Check sheet for the modelled part. Datum: model origin and axes. Units: mm. Face numbers are marked on the shaded views. Coordinates: 2 decimals unless noted, no trailing zeros. Loops run counter-clockwise (first coordinate to the right, second up) from the corner with the lowest first, then second, coordinate; pieces in that order, holes last. Notation, with made-up numbers: M 10,4 L 25,4 A27 cw 25,34 Z; hole C 37,-39.75 d7. An arc over 180 degrees is marked long. Use CSV: the item, a comma, the result in double quotes. Start each with the question number.
(1) Section check C-C on y = 61. Record the cut outline in (x, z), and give its area (3 significant figures).
(2) Section check A-A on z = 0. Record the cut outline in (x, y), and give its area (3 significant figures).
(3) Draft check along X on the marked faces 1, 2 and 3. Enter one of: pulls with the +X half, pulls with the -X half, needs draft (parallel to the pull), parting line crosses it, or undercut.
(4) Go/stop test with flat-tipped pins: pin 1 Ø4 at (y, z) = (-13.5, -33) entering from -X; pin 2 Ø4 at (y, z) = (-46, 34.5) entering from -X; pin 3 Ø4 at (y, z) = (-39.5, 39) entering from +X. Record where each tip stops, or that it passes through.
(5) Scan lines: line 1 (Z direction, x = 0, y = 8); line 2 (Z direction, x = -20, y = 9.5). Record each from-to range of solid material in increasing order.
(6) Section check B-B on x = 0. Record the cut outline in (y, z), and give its area (3 significant figures).
Autodesk Inventor part; units mm, degrees
ref_plane "YZ Plane" through (0, 0, 0) normal (1, 0, 0) x (0, 1, 0)
ref_plane "XZ Plane" through (0, 0, 0) normal (0, 1, 0) x (-1, 0, 0)
ref_plane "XY Plane" through (0, 0, 0) normal (0, 0, 1) x (1, 0, 0)
sketch "Sketch1" plane through (0, 0, 0) normal (0, 0, 1) x (1, 0, 0)
  line L0 (-50, 88.8965) -> (-25, 88.8965)
  line L1 (-25, 88.8965) -> (-25, -61.1035)
  line L2 (-25, -61.1035) -> (-50, -61.1035)
  line L3 (-50, -61.1035) -> (-50, 88.8965)
  line L4 (0, 88.8965) -> (0, -88.8965)
  point P0 (0, 0)
  point P1 (0, 0)
  dimension "d10" = 150
  dimension "d12" = 25
  dimension "d13" = 50
revolve "Revolution1" add sketch "Sketch1" angle 360 about axis through (0, 88.8965, 0) along (0, -1, 0)
chamfer "Chamfer1" distance 2 angle 45 2 edges at (25, 88.8965, 0) (25, -61.1035, 0)
chamfer "Chamfer3" distance 5 angle 45 2 edges at (50, 88.8965, 0) (50, -61.1035, 0)
properties part number "TestPart"
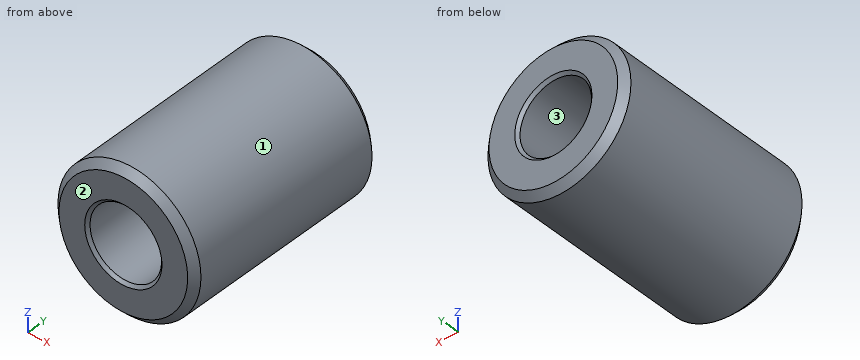
Outcome:
1,outline,"C 0,0 d100; hole C 0,0 d50"
1,area,"5,890 mm²"
2,outline,"M -50,-56.1 L -45,-61.1 L -27,-61.1 L -25,-59.1 L -25,86.9 L -27,88.9 L -45,88.9 L -50,83.9 Z; M 25,-59.1 L 27,-61.1 L 45,-61.1 L 50,-56.1 L 50,83.9 L 45,88.9 L 27,88.9 L 25,86.9 Z"
2,area,"7,440 mm²"
3,face 1,"parting line crosses it"
3,face 2,"needs draft"
3,face 3,"undercut"
4,pin 1,"stops at x = -39.23"
4,pin 2,"stops at x = -38"
4,pin 3,"stops at x = 33.63"
5,line 1,"z = -50 to -25, 25 to 50"
5,line 2,"z = -45.83 to -15, 15 to 45.83"
6,outline,"M -61.1,-45 L -56.1,-50 L 83.9,-50 L 88.9,-45 L 88.9,-27 L 86.9,-25 L -59.1,-25 L -61.1,-27 Z; M -61.1,27 L -59.1,25 L 86.9,25 L 88.9,27 L 88.9,45 L 83.9,50 L -56.1,50 L -61.1,45 Z"
6,area,"7,440 mm²"
